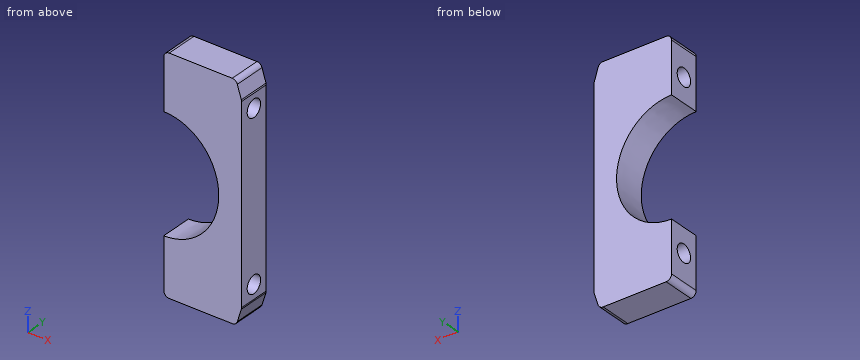
```python
from build123d import *

# Parameters (mm, degrees)
EXTRUDE_1_DEPTH     = 12
FILLET_1_R          = 2
FILLET_2_R          = 2
SKETCH_2_R          = 3.25
CUT_EXTRUDE_1_DEPTH = 53.832281956


with BuildPart() as part:
    # 草圖1 → 填料-伸長1 (new body)
    with BuildSketch(Plane(origin=(0, 0, 0), x_dir=(1, 0, 0), z_dir=(0, 1, 0))):
        with BuildLine():
            Line((0, 21.5), (0, 42.5))
            Line((0, 42.5), (27, 42.5))
            Line((27, 42.5), (29, 36))
            Line((29, 36), (29, -36))
            Line((29, -36), (27, -42.5))
            Line((27, -42.5), (0, -42.5))
            Line((0, -42.5), (0, -21.5))
            add(Edge.make_bspline(
                [(0, -21.5), (20.5, -21.5), (20.5, 0), (20.5, 21.5), (0, 21.5)],
                knots=[3.141592654, 3.141592654, 3.141592654, 4.71238898, 4.71238898, 6.283185307, 6.283185307, 6.283185307], degree=2, weights=[1, 0.707106781, 1, 0.707106781, 1]))
        make_face()
    extrude(amount=EXTRUDE_1_DEPTH)

    # 圓角1
    fillet_1_edges = [part.edges().sort_by_distance(p)[0] for p in [
        (29, 6, 36),
        (27, 6, 42.5),
    ]]
    fillet(fillet_1_edges, radius=FILLET_1_R)

    # 圓角2
    fillet_2_edges = [part.edges().sort_by_distance(p)[0] for p in [
        (0, 6, -42.5),
        (27, 6, -42.5),
        (29, 6, -36),
        (0, 6, 42.5),
    ]]
    fillet(fillet_2_edges, radius=FILLET_2_R)

    # 草圖2 → 除料-伸長1 (cut, through all)
    with BuildSketch(Plane(origin=(29, 0, 0), x_dir=(0, 0, -1), z_dir=(1, 0, 0))):
        with Locations((30.5, 6)):
            Circle(SKETCH_2_R)
        with Locations(Location((-30.5, 6, 0), (0, 0, 180))):
            Circle(SKETCH_2_R)
    extrude(amount=-CUT_EXTRUDE_1_DEPTH, mode=Mode.SUBTRACT)


solid = part.part
```
Can you work these out from the model? Positions are in its coordinate system, mm. Coordinates: 2 decimals unless noted, no trailing zeros. Loops run counter-clockwise (first coordinate to the right, second up) from the corner with the lowest first, then second, coordinate; pieces in that order, holes last. Notation, with made-up numbers: (42.5, 9) -> (68.5, 9) arc R27 cw to (68.5, 38) -> close; hole circle Ø2 at (34, -2.5). An arc over 180 degrees is marked (long way). Answer as a JSON object with one key per item and string values.
1) Imagine slicing it at B-B (x = 22.5). Please give me the cut outline in (y, z), then the cut area to 3 significant figures.
Results:
{"outline": "(0, -42.5) -> (12, -42.5) -> (12, 42.5) -> (0, 42.5) -> close; hole circle Ø6.5 at (6, -30.5); hole circle Ø6.5 at (6, 30.5)", "area": "954 mm^2"}
2) For P1, Ø5, axis at y = 6, z = 30.5, coming from the +X side, with a flat end and sliding along its axis, tell me the tip position at first contact or that it passes through.
Results:
{"P1": "passes through"}
3) If I drill on line 1 (Y direction, x = 14.5, z = -30.5); line 2 (Z direction, x = 21.5, y = 5.5); line 3 (Z direction, x = 24, y = 8), over which ranges is the centre line in solid material (lowest first)?
Results:
{"line 1": "y = 0 to 2.75, 9.25 to 12", "line 2": "z = -42.5 to -33.71, -27.29 to 27.29, 33.71 to 42.5", "line 3": "z = -42.5 to -33.06, -27.94 to 27.94, 33.06 to 42.5"}
4) Imagine slicing it at A-A (z = 30.5). Please give me the cut outline in (x, y).
Results:
{"outline": "(0, 0) -> (29, 0) -> (29, 2.75) -> (0, 2.75) -> close; (0, 9.25) -> (29, 9.25) -> (29, 12) -> (0, 12) -> close"}
5) Imagine slicing it at C-C (y = 6). Count the separate pieces of the cut face and the enclosed holes in it, then the cut area to 3 significant figures.
Results:
{"separate pieces": "3", "enclosed holes": "0", "area": "1,380 mm^2"}
